from build123d import *

# Parameters (mm, degrees)
SKETCH2_W                = 50
SKETCH2_H                = 18
BOSS_EXTRUDE1_DEPTH      = 60
CUT_EXTRUDE1_DEPTH       = 50
SKETCH4_R                = 16
BOSS_EXTRUDE2_DEPTH      = 11
SKETCH5_R                = 15
BOSS_EXTRUDE3_DEPTH      = 10
SKETCH6_R                = 4
CUT_EXTRUDE2_DEPTH       = 45
FILLET1_R                = 7
FILLET6_R                = 7
SKETCH7_W                = 10
SKETCH7_H                = 5
BOSS_EXTRUDE4_DEPTH      = 12
SKETCH8_R                = 2.017979808
CUT_EXTRUDE3_DEPTH       = 10
CUT_EXTRUDE4_DEPTH       = 10
BOSS_EXTRUDE5_DEPTH      = 4
BOSS_EXTRUDE6_DEPTH      = 6
BOSS_EXTRUDE6_DEPTH_BACK = 73
SKETCH12_R               = 2.5
SKETCH15_W               = 6.308184524
SKETCH15_H               = 0.262670096
CUT_EXTRUDE6_DEPTH       = 0.5
BOSS_EXTRUDE7_DEPTH      = 55
SKETCH22_R               = 8.328168783
BOSS_EXTRUDE8_DEPTH      = 3
SKETCH23_R               = 2.62195597
BOSS_EXTRUDE9_DEPTH      = 2
FILLET7_R                = 2
FILLET8_R                = 1
BOSS_EXTRUDE10_DEPTH     = 2
SKETCH25_R               = 1.5
CUT_EXTRUDE7_DEPTH       = 2
SKETCH27_W               = 12.756486499
SKETCH27_H               = 4.738083454
BOSS_EXTRUDE11_DEPTH     = 14
SKETCH28_R               = 2
CUT_EXTRUDE8_DEPTH       = 14


with BuildPart() as part:
    # Sketch2 → Boss-Extrude1 (new body)
    with BuildSketch(Plane.XY):
        Rectangle(SKETCH2_W, SKETCH2_H)
    extrude(amount=-BOSS_EXTRUDE1_DEPTH)

    # Sketch3 → Cut-Extrude1 (cut)
    with BuildSketch(Plane(origin=(0, 9, 0), x_dir=(1, 0, 0), z_dir=(0, 1, 0))):
        with BuildLine():
            Line((0, 55), (0, 60))
            Line((0, 60), (-25, 60))
            Line((-25, 60), (-25, 30))
            ThreePointArc((-25, 30), (-17.67766953, 47.67766953), (0, 55))
        make_face()
        with BuildLine():
            Line((25, 60), (0, 60))
            Line((0, 60), (0, 55))
            ThreePointArc((0, 55), (17.67766953, 47.67766953), (25, 30))
            Line((25, 30), (25, 60))
        make_face()
    extrude(amount=-CUT_EXTRUDE1_DEPTH, mode=Mode.SUBTRACT)

    # Sketch4 → Boss-Extrude2 (add)
    with BuildSketch(Plane(origin=(0, 9, 0), x_dir=(1, 0, 0), z_dir=(0, 1, 0))):
        with Locations(Location((0, 30, 0), (0, 0, 270))):
            Circle(SKETCH4_R)
    extrude(amount=BOSS_EXTRUDE2_DEPTH)

    # Sketch5 → Boss-Extrude3 (add)
    with BuildSketch(Plane(origin=(0, 20, 0), x_dir=(1, 0, 0), z_dir=(0, 1, 0))):
        with Locations(Location((0, 30, 0), (0, 0, 270))):
            Circle(SKETCH5_R)
    extrude(amount=BOSS_EXTRUDE3_DEPTH)

    # Sketch6 → Cut-Extrude2 (cut)
    with BuildSketch(Plane(origin=(0, 30, 0), x_dir=(1, 0, 0), z_dir=(0, 1, 0))):
        with Locations(Location((0, 30, 0), (0, 0, 270))):
            Circle(SKETCH6_R)
    extrude(amount=-CUT_EXTRUDE2_DEPTH, mode=Mode.SUBTRACT)

    # Fillet1
    fillet1_edges = [part.edges().sort_by_distance(p)[0] for p in [
        (0, 9, 0),
    ]]
    fillet(fillet1_edges, radius=FILLET1_R)

    # Fillet6
    # the kernel refuses this fillet: 7 mm, written as the material it takes off along each edge
    with BuildSketch(Plane(origin=(-25, 9, 10.5), x_dir=(0, -1, 0), z_dir=(0, 0, -1))) as fillet6_piece_1:
        with BuildLine():
            CenterArc((FILLET6_R, -FILLET6_R), FILLET6_R, 90, 90)
            Line((0, -FILLET6_R), (0, 0))
            Line((0, 0), (FILLET6_R, 0))
        make_face()
    extrude(amount=40.5, mode=Mode.SUBTRACT)
    with BuildSketch(Plane(origin=(0, 9, -30), x_dir=(-1, 0, 0), z_dir=(0, 0, 1))) as fillet6_piece_2:
        with BuildLine():
            CenterArc((25 - FILLET6_R, FILLET6_R), FILLET6_R, 270, 90)
            Line((25, FILLET6_R), (25, 0))
            Line((25, 0), (25 - FILLET6_R, 0))
        make_face()
    revolve(axis=Axis((0, 9, -30), (0, -1, 0)), revolution_arc=180, mode=Mode.SUBTRACT)
    with BuildSketch(Plane(origin=(25, 9, 10.5), x_dir=(0, -1, 0), z_dir=(0, 0, -1))) as fillet6_piece_3:
        with BuildLine():
            CenterArc((FILLET6_R, FILLET6_R), FILLET6_R, 180, 90)
            Line((0, FILLET6_R), (0, 0))
            Line((0, 0), (FILLET6_R, 0))
        make_face()
    extrude(amount=40.5, mode=Mode.SUBTRACT)

    # Sketch7 → Boss-Extrude4 (add)
    with BuildSketch(Plane(origin=(25, 0, 0), x_dir=(0, 0, -1), z_dir=(1, 0, 0))):
        with Locations((15, -4.5)):
            Rectangle(SKETCH7_W, SKETCH7_H)
    extrude(amount=BOSS_EXTRUDE4_DEPTH)

    # Sketch8 → Cut-Extrude3 (cut)
    with BuildSketch(Plane(origin=(0, -7, 0), x_dir=(-1, 0, 0), z_dir=(0, -1, 0))):
        with Locations(Location((-33, 15, 0), (0, 0, 90))):
            Circle(SKETCH8_R)
    extrude(amount=-CUT_EXTRUDE3_DEPTH, mode=Mode.SUBTRACT)

    # Sketch9 → Cut-Extrude4 (cut)
    with BuildSketch(Plane.XZ.offset(7)):
        with BuildLine():
            Line((37, -20), (37, -15.487118702))
            add(Edge.make_bspline(
                [(29.301025402, -20), (31.159014878, -19.577955894), (35.343998587, -19.634790074), (36.930791765, -16.465392679), (37, -15.487118702)],
                knots=[0, 0, 0, 0, 0.665986255, 0.952522337, 0.952522337, 0.952522337, 0.952522337], degree=3))
            Line((29.301025402, -20), (37, -20))
        make_face()
        with BuildLine():
            Line((37, -10), (29.301025402, -10))
            add(Edge.make_bspline(
                [(29.301025402, -10), (31.159014878, -10.422044106), (35.343998587, -10.365209926), (36.930791765, -13.534607321), (37, -14.512881298)],
                knots=[0, 0, 0, 0, 0.665986255, 0.952522337, 0.952522337, 0.952522337, 0.952522337], degree=3))
            Line((37, -14.512881298), (37, -10))
        make_face()
    extrude(amount=-CUT_EXTRUDE4_DEPTH, mode=Mode.SUBTRACT)

    # Sketch10 → Boss-Extrude5 (add)
    with BuildSketch(Plane(origin=(25, 0, 0), x_dir=(0, 0, -1), z_dir=(1, 0, 0))):
        Polygon((7.181671506, 1.449117939), (2.565182327, 1.302963931), (0.383510821, -2.768109978), (2.818328494, -6.693029879), (7.434817673, -6.546875871), (9.616489179, -2.475801962), align=None)
    extrude(amount=BOSS_EXTRUDE5_DEPTH)

    # Sketch12 → Boss-Extrude6 (add, two sides: drawn at the far end of the back side and taken through both)
    with BuildSketch(Plane(origin=(29, 0, 0), x_dir=(0, 0, -1), z_dir=(1, 0, 0)).offset(-BOSS_EXTRUDE6_DEPTH_BACK)):
        with Locations((5, -2.62195597)):
            Circle(SKETCH12_R)
    extrude(amount=BOSS_EXTRUDE6_DEPTH + BOSS_EXTRUDE6_DEPTH_BACK)

    # Sketch15 → Cut-Extrude6 (cut)
    with BuildSketch(Plane(origin=(35, 0, 0), x_dir=(0, 0, -1), z_dir=(1, 0, 0))):
        with Locations((5, -2.62195597)):
            Rectangle(SKETCH15_W, SKETCH15_H)
    extrude(amount=-CUT_EXTRUDE6_DEPTH, mode=Mode.SUBTRACT)

    # Sketch16 → Boss-Extrude7 (add)
    with BuildSketch(Plane.ZY.offset(25)):
        with BuildLine():
            Line((-5, 14.87804403), (12.5, -2.62195597))
            ThreePointArc((12.5, -2.62195597), (7.374368671, -14.996324641), (-5, -20.12195597))
            Line((-5, -20.12195597), (-22.5, -2.62195597))
            ThreePointArc((-22.5, -2.62195597), (-17.374368671, 9.752412701), (-5, 14.87804403))
        make_face()
    extrude(amount=BOSS_EXTRUDE7_DEPTH)

    # Sketch22 → Boss-Extrude8 (add)
    with BuildSketch(Plane.ZY.offset(80)):
        with Locations((-5, -2.62195597)):
            Circle(SKETCH22_R)
    extrude(amount=BOSS_EXTRUDE8_DEPTH)

    # Sketch23 → Boss-Extrude9 (add)
    with BuildSketch(Plane.ZY.offset(83)):
        with Locations((-5, -2.62195597)):
            Circle(SKETCH23_R)
    extrude(amount=BOSS_EXTRUDE9_DEPTH)

    # Fillet7
    fillet7_edges = [part.edges().sort_by_distance(p)[0] for p in [
        (-83, -2.62195597, -13.328168783),
    ]]
    fillet(fillet7_edges, radius=FILLET7_R)

    # Fillet8
    fillet8_edges = [part.edges().sort_by_distance(p)[0] for p in [
        (-85, -2.62195597, -7.62195597),
    ]]
    fillet(fillet8_edges, radius=FILLET8_R)

    # Sketch24 → Boss-Extrude10 (add)
    with BuildSketch(Plane(origin=(-25, 0, 0), x_dir=(0, 0, -1), z_dir=(1, 0, 0))):
        with BuildLine():
            Line((-13.980304455, -2.688046863), (5.159392937, 16.451650529))
            Line((5.159392937, 16.451650529), (20.658441278, 16.451650529))
            ThreePointArc((20.658441278, 16.451650529), (22.779761622, 15.572970872), (23.658441278, 13.451650529))
            Line((23.658441278, 13.451650529), (23.658441278, -2.877728254))
            Line((23.658441278, -2.877728254), (5.255772284, -21.280397249))
            Line((5.255772284, -21.280397249), (-10.980304455, -21.280397249))
            ThreePointArc((-10.980304455, -21.280397249), (-13.101624798, -20.401717592), (-13.980304455, -18.280397249))
            Line((-13.980304455, -18.280397249), (-13.980304455, -2.688046863))
        make_face()
    extrude(amount=BOSS_EXTRUDE10_DEPTH)

    # Sketch25 → Cut-Extrude7 (cut)
    with BuildSketch(Plane.ZY.offset(25)):
        with Locations((-20.658441278, 13.451650529)):
            Circle(SKETCH25_R)
        with Locations(Location((11.073606499, -18.280397249, 0), (0, 0, 180))):
            Circle(SKETCH25_R)
    extrude(amount=-CUT_EXTRUDE7_DEPTH, mode=Mode.SUBTRACT)

    # Sketch27 → Boss-Extrude11 (add)
    with BuildSketch(Plane.XY):
        with Locations((-16.621756751, -3.512365056)):
            Rectangle(SKETCH27_W, SKETCH27_H)
    extrude(amount=BOSS_EXTRUDE11_DEPTH)

    # Sketch28 → Cut-Extrude8 (cut)
    with BuildSketch(Plane(origin=(0, -5.881406783, 0), x_dir=(-1, 0, 0), z_dir=(0, -1, 0))):
        with BuildLine():
            add(Edge.make_bspline(
                [(23, -13.980304455), (21.040358256, -13.849946774), (18.327335378, -12.869508638), (14.76618265, -13.383152912), (13.195630898, -12.157690347), (12.453642875, -10.967120732), (11.825664424, -9.487701946), (11.427276145, -7.580341481), (11.452990141, -5.432672222), (11.129880797, -2.792351119), (11.084820543, -0.923222192), (10.243513501, 0)],
                knots=[0, 0, 0, 0, 0.253392468, 0.384448091, 0.437710576, 0.505134134, 0.567821926, 0.648624813, 0.759593973, 0.849288238, 1, 1, 1, 1], degree=3))
            Line((10.243513501, 0), (10.243513501, -14))
            Line((10.243513501, -14), (23, -14))
            Line((23, -14), (23, -13.980304455))
        make_face()
        with Locations(Location((16.62175675, -10.436159793, 0), (0, 0, 90))):
            Circle(SKETCH28_R)
    extrude(amount=-CUT_EXTRUDE8_DEPTH, mode=Mode.SUBTRACT)


solid = part.part
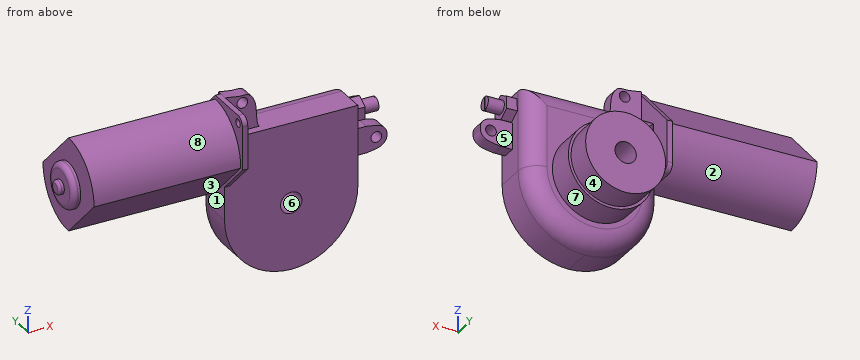
Can you work these out from the model? Positions are in its coordinate system, mm. Face numbers are marked on the shaded views. A direction names the side the tool comes from. Give positions to 0.01 mm unless a question says otherwise; leave off trailing zeros. Loops run counter-clockwise (first coordinate to the right, second up) from the corner with the lowest first, then second, coordinate; pieces in that order, holes last. Notation, with made-up numbers: M 47.25,28 L 67.25,28 A30 cw 67.25,55 Z; hole C 12,7.5 d7. An arc over 180 degrees is marked long. One line per item, written item: value.
1) On a 3-axis mill with a long thin cutter (end or side, diameter ignored), from which of +Z, -Z, +X, -X, +Y, -Y can I reach the whole of each face in a straight line? I mean the marked faces 1, 2, 3 and 4. Say none if no direction works.
Geometry check:
face 1: -X
face 2: -Z, -X, +Y
face 3: -Z, -X, -Y
face 4: +Y
2) Imagine slicing it at A-A on x = 27.5. Write out the boundary of the cut face in (y, z), and give its area (3 significant figures).
Geometry check:
outline: M -7,-20 L -2,-20 L -2,-10 L -7,-10 Z; M -6.69,-2.82 L -6.55,-7.43 L -2.48,-9.62 L 1.45,-7.18 L 1.3,-2.57 L -2.77,-0.38 Z
area: 105 mm²
3) I'm going to push flat-ended pins straight in: pin 1 (12 mm diameter, centred on x = 0.5, y = 17.5, fed in from -Z); pin 2 (11 mm diameter, centred on x = 31, z = -14.5, fed in from -Y); pin 3 (4 mm diameter, centred on y = -18.28, z = 11.07, fed in from +X); pin 4 (13 mm diameter, centred on x = 0, z = -30, fed in from +Y). Where does each tip first touch, or does it pass through?
Geometry check:
pin 1: stops at z = -46
pin 2: stops at y = -7
pin 3: stops at x = -23
pin 4: stops at y = 30
4) Imagine slicing it at B-B on y = 25. Write out the boundary of the cut face in (x, z).
Geometry check:
outline: C 0,-30 d30; hole C 0,-30 d8
5) Imagine slicing it at C-C on x = -56.5. Write out the boundary of the cut face in (y, z).
Geometry check:
outline: M -20.12,-5 L -2.62,-22.5 A17.5 ccw 14.88,-5 L -2.62,12.5 A17.5 ccw Z
6) Thinking about a two-plate mould opening in Z: for the marked faces 5, 6, 7 and 8, which applies, +Z half, -Z half, draft (parallel to the pull), parting line (faces both ways), or undercut?
Geometry check:
face 5: draft
face 6: undercut
face 7: parting line
face 8: +Z half
7) Please list where these lines run through material, in increasing order: line 1 (Y direction, x = 12.5, z = -28.5); line 2 (Y direction, x = -11, z = -40.5); line 3 (X direction, y = 4, z = -30).
Geometry check:
line 1: y = -9 to 30
line 2: y = -9 to 20
line 3: x = -24.71 to -4, 4 to 24.71
